Verification items for the finished model (mm, model axes). Face numbers are marked on the shaded views. A direction names the side the tool comes from. Give positions to 0.01 mm unless a question says otherwise; leave off trailing zeros. Write each loop counter-clockwise with the first axis right and the second up, starting at its lowest first coordinate (ties: lowest second). Pieces come first, ordered by that corner, then holes. Notation, with made-up numbers: M -10,49 L 36,49 A12 cw 36,70 Z; hole C 45,14.5 d11. An arc over 180 degrees is marked long. Answer as a JSON object with one key per item and string values.
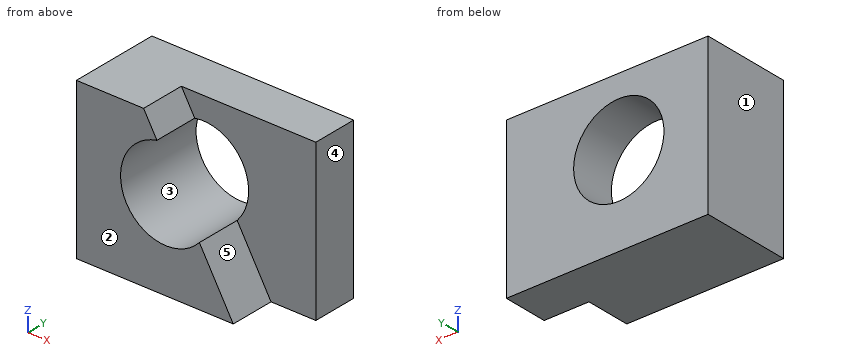
```python
from build123d import *

# Parameters (mm, degrees)
F0_W     = 57.15
F0_H     = 44.45
F1_DEPTH = 25.4
F2_R     = 12.793463
F3_DEPTH = 25.4
F4_W     = 12.7
F4_H     = 12.7
F5_DEPTH = 44.45
F7_DEPTH = 12.7


with BuildPart() as f1:
    # F0 (on Front) → F1 (new body)
    with BuildSketch(Plane.XZ):
        with Locations((-37.38983, 36.408463)):
            Rectangle(F0_W, F0_H)
    extrude(amount=F1_DEPTH)

    # F2 (on face) → F3 (cut)
    with BuildSketch(Plane.XZ.offset(25.4)):
        with Locations((-40.658294, 39.49)):
            Circle(F2_R)
    extrude(amount=-F3_DEPTH, mode=Mode.SUBTRACT)

    # F4 (on face) → F5 (cut)
    with BuildSketch(Plane.XY.offset(58.633463)):
        with Locations((-15.16483, -19.05)):
            Rectangle(F4_W, F4_H)
    extrude(amount=-F5_DEPTH, mode=Mode.SUBTRACT)

    # F6 (on face) → F7 (cut)
    with BuildSketch(Plane.XZ.offset(25.4)):
        Polygon((-21.51483, 58.633463), (-46.91483, 58.633463), (-21.51483, 14.183463), align=None)
    extrude(amount=-F7_DEPTH, mode=Mode.SUBTRACT)


solid = f1.part
```
1) Access from +Z, -Z, +X, -X, +Y, -Y to the whole of each face (thin tool, end or side, straight path). Record for the marked faces 4 and 5.
Completed:
{"face 4": "+Z, -Z, +X, +Y, -Y", "face 5": "+Z, +X, -Y"}
2) Release check for a two-part mould opening along X. For the marked faces 1, 2 and 3 record: pulls with the +X half, pulls with the -X half, needs draft (parallel to the pull), parting line crosses it, or undercut.
Completed:
{"face 1": "pulls with the -X half", "face 2": "needs draft", "face 3": "undercut"}
3) Section check A-A on z = 39.49. Record the boundary of the cut face in (x, y), and give its area (3 significant figures).
Completed:
{"outline": "M -65.96,-25.4 L -53.45,-25.4 L -53.45,0 L -65.96,0 Z; M -27.86,-12.7 L -8.81,-12.7 L -8.81,0 L -27.86,0 Z", "area": "560 mm2"}
4) Go/stop test with flat-tipped pins: pin 1 (6 mm diameter, centred on x = -17.5, z = 51.5, fed in from +Y); pin 2 (11.5 mm diameter, centred on x = -32.5, z = 45.5, fed in from -Y); pin 3 (20.5 mm diameter, centred on x = -40.66, z = 39.49, fed in from +Y). Record where each tip stops, or that it passes through.
Completed:
{"pin 1": "stops at y = 0", "pin 2": "stops at y = -12.7", "pin 3": "passes through"}
5) Thickness scan on L1, parallel to X at y = -9, z = 39.49; L2, parallel to Y at x = -13.5, z = 39; L3, parallel to X at y = -5, z = 31.5. Record the ranges inside material, lowest first.
Completed:
{"L1": "x = -65.96 to -53.45, -27.86 to -8.81", "L2": "y = -12.7 to 0", "L3": "x = -65.96 to -50.65, -30.67 to -8.81"}
6) Section check C-C on y = -10. Record the boundary of the cut face in (x, z).
Completed:
{"outline": "M -65.96,14.18 L -8.81,14.18 L -8.81,58.63 L -65.96,58.63 Z; hole C -40.66,39.49 d25.59"}
7) Section check D-D on y = -23.25. Record the boundary of the cut face in (x, z), and give its area (3 significant figures).
Completed:
{"outline": "M -65.96,14.18 L -21.51,14.18 L -31.11,30.98 A12.79 cw long -43.15,52.04 L -46.91,58.63 L -65.96,58.63 Z", "area": "1,050 mm2"}
8) Section check B-B on x = -29. Record the boundary of the cut face in (y, z).
Completed:
{"outline": "M -25.4,14.18 L 0,14.18 L 0,34.22 L -12.7,34.22 L -12.7,27.28 L -25.4,27.28 Z; M -12.7,44.76 L 0,44.76 L 0,58.63 L -12.7,58.63 Z"}
